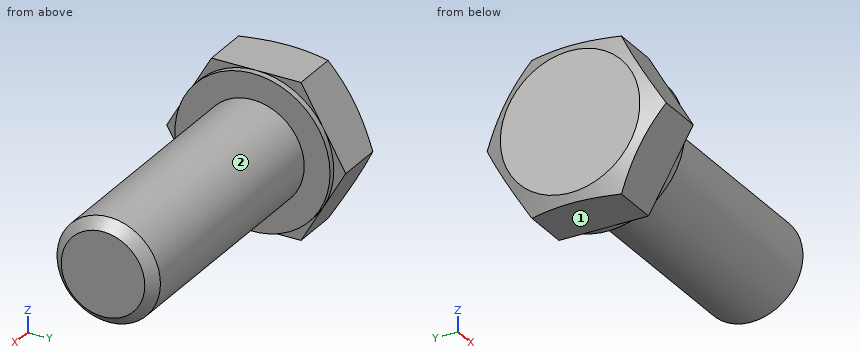
Autodesk Inventor part; units mm, degrees
ref_plane "Work Plane1" through (1.525, 0, 0) normal (0, 0, 1) x (1, 0, 0)
ref_plane "YZ Plane" through (0, 0, 0) normal (1, 0, 0) x (0, 1, 0)
ref_plane "XZ Plane" through (0, 0, 0) normal (0, 1, 0) x (-1, 0, 0)
sketch "Эскиз1" plane through (0, 0, 0) normal (0, 0, 1) x (1, 0, 0)
  line L0 (0, 6) -> (0, 4)
  line L1 (1.25, 4) -> (20, 4)
  line L2 (20, 4) -> (20, 0)
  line L3 (20, 0) -> (-0.5001, 0)
  line L4 (-4.6001, 0) -> (24.1, 0)
  line L5 (-0.5001, 0) -> (-0.5001, 6)
  line L6 (-0.5001, 6) -> (0, 6)
  line L7 (1.25, 4) -> (0.4831, 4)
  line L8 (0.4831, 4) -> (0, 4)
  line L9 (0, -1.2) -> (0, 7.2)
  dimension "d0" = 20
  dimension "d1" = 18.75
  dimension "d2" = 8
  dimension "d9" = 0.5001
  dimension "d10" = 12
  dimension "d13" = 0.7669
  dimension "d14" = 8
revolve "Базовый элемент" add sketch "Эскиз1" angle 360 about axis through (20, 0, 0) along (-1, 0, 0)
sketch "Эскиз2" plane through (-0.5001, 0, 0) normal (-1, 0, 0) x (0, 0, 1)
  line L0 (0, 6.9282) -> (6, 3.4641)
  line L1 (6, 3.4641) -> (6, -3.4641)
  line L2 (6, -3.4641) -> (0, -6.9282)
  line L3 (0, -6.9282) -> (-6, -3.4641)
  line L4 (-6, -3.4641) -> (-6, 3.4641)
  line L5 (-6, 3.4641) -> (0, 6.9282)
  point P0 (0, 0)
  point P1 (0, 0)
  dimension "d11" = 12
extrude "С головкой" add sketch "Эскиз2" along normal blind 4.5
sketch "Эскиз4" plane through (0, 0, 0) normal (0, 0, 1) x (1, 0, 0)
  line L0 (-5.0001, 5.4) -> (-5.0001, 6.9282)
  line L1 (-5.0001, 6.9282) -> (-4.1178, 6.9282)
  line L2 (-4.1178, 6.9282) -> (-5.0001, 5.4)
  line L3 (-5.9001, 0) -> (0.3999, 0)
  line L4 (-0.5001, 6.9282) -> (-5.0001, 6.9282)
  line L5 (-5.0001, 3.4641) -> (-5.0001, 6.9282)
  dimension "d5" = 30
  dimension "d19" = 10.8
revolve "Фаска1" cut sketch "Эскиз4" angle 360 about axis through (-10, 0, 0) along (1, 0, 0)
thread "Резьба"
chamfer "Фаска2" distance 0.7668 distance2 0.7669 1 edges at (20, -4, 0) measured on face at (20, 1.3194, 0.8842)
ref_plane "Work Plane1" through (1.525, 0, 0) normal (0, 0, 1) x (1, 0, 0)
equation "\"d0\" = NLG"
equation "\"d1\" = GEL"
equation "\"d2\" = GD"
equation "\"d10\" = SD2"
equation "\"d14\" = BDM"
equation "\"d11\" = SW"
equation "\"d3\" = KOH - SD"
equation "\"d5\" = ANG1"
equation "\"d19\" = SW0"
equation "\"d15\" = GEL"
equation "\"d6\" = -0.5 * SPD + 0.5 * GD"
equation "\"NLG\" = 20"
equation "\"GD\" = NND"
equation "\"BDM\" = NND"
equation "\"KOH\" = 5"
equation "\"GEL\" = 18.75"
equation "\"SW\" = 12"
equation "\"SW0\" = 10.8"
equation "\"SPD\" = NND - 1.2269 * PTC"
equation "\"SD2\" = SW"
equation "\"SD\" = 0.5"
equation "\"ANG1\" = 30deg"
equation "\"GAL\" = 0.61345 * PTC"
equation "\"GUL\" = 0.61345 * PTC"
equation "\"RR\" = 0.1"
equation "\"GD1\" = THREADDIA - 1.2269 * PTC"
equation "\"THREADDIA\" = 8"
equation "\"TOA\" = 30deg"
equation "\"PTC\" = 1.25"
equation "\"NND\" = 8"
equation "\"E0\" = 1.155 * SW"
properties part number "Болт M8-6gx20 ГОСТ 7808-70" material "Сталь, мягкая"
Geometry: final body of the model. Coordinates: model frame, mm. Face numbers are marked on the shaded views. A direction names the side the tool comes from. Give positions to 0.01 mm unless a question says otherwise; leave off trailing zeros. Write each loop counter-clockwise with the first axis right and the second up, starting at its lowest first coordinate (ties: lowest second). Pieces come first, ordered by that corner, then holes.
(1) Ray query, line 1 (X direction, y = 2.5, z = 4.25); line 2 (Z direction, x = 19, y = -2). Return the intervals inside material, ascending.
(2) First-contact query: P1, Ø0.9, axis at y = 1.5, z = 5, coming from the +X side; P2, Ø2.5, axis at y = -1.5, z = 4.5, coming from the +X side; P3, Ø1, axis at x = 3.5, z = 1.5, coming from the -Y side. Flat tips, straight axial feed; report the tip coordinate or a pass-through.
(3) Cut plane B-B, the plane x = 0.75. Return loops of the section in (y, z).
(4) Access query for the marked faces 1 and 2. Directions: +Z, -Z, +X, -X, +Y, -Y. A direction counts if a zero-diameter tool reaches every point of the face in a straight line with its end or side. Return the directions, or none.
(5) Cut plane A-A, the plane x = -3.5. Return loops of the section in (y, z), then the cut area to 3 significant figures.
Values follow:
1. line 1: x = -5 to 0
1. line 2: z = -3.46 to 3.46
2. P1: stops at x = 0
2. P2: stops at x = 19.74
2. P3: stops at y = -3.87
3. outline: circle Ø8 at (0, 0)
4. face 1: -Z, +X, -X, +Y, -Y
4. face 2: +X
5. outline: (-6.93, 0) - (-3.46, -6) - (3.46, -6) - (6.93, 0) - (3.46, 6) - (-3.46, 6) - close
5. area: 125 mm2
